from build123d import *

# Parameters (mm, degrees)
F1_DEPTH = 20


with BuildPart() as f1:
    # F0 (on Front) → F1 (new body)
    with BuildSketch(Plane.XZ):
        with BuildLine():
            Line((550, 0), (50, 0))
            ThreePointArc((50, 0), (14.644661, -14.644661), (0, -50))
            Line((0, -50), (0, -650))
            ThreePointArc((0, -650), (14.644661, -685.355339), (50, -700))
            Line((50, -700), (296.851258, -700))
            ThreePointArc((296.851258, -700), (317.85788, -695.37314), (334.976714, -682.348872))
            Line((334.976714, -682.348872), (588.125457, -383.994997))
            ThreePointArc((588.125457, -383.994997), (596.93758, -368.875855), (600, -351.646125))
            Line((600, -351.646125), (600, -50))
            ThreePointArc((600, -50), (585.355339, -14.644661), (550, 0))
        make_face()
    extrude(amount=F1_DEPTH)


solid = f1.part
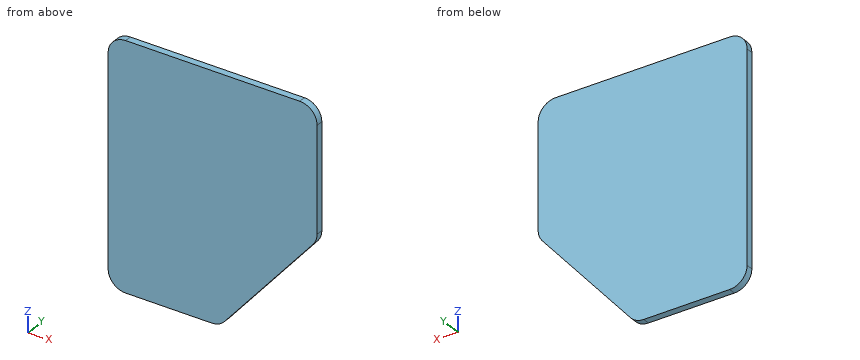
Verification items for the finished model (mm, model axes). Round coordinates to 2 decimals unless told otherwise and drop trailing zeros. Loops run counter-clockwise (first coordinate to the right, second up) from the corner with the lowest first, then second, coordinate; pieces in that order, holes last. Notation, with made-up numbers: (48, 67) - (69, 67) arc R14 cw to (69, 77) - close; hole circle Ø5 at (1.25, 58). An arc over 180 degrees is marked (long way). Answer in a Markdown table with one row per item. Add a question column.
Q1. Section check C-C on z = -565. Enter the section's corners in (x, y).
Q2. Section check A-A on y = -6.75. Enter the section's corners in (x, z) (3 decimals), plus the area to 3 significant figures.
Q3. Material ranges on line 1 (Z direction, x = 298, y = -1); line 2 (X direction, y = -17.5, z = -476); line 3 (Z direction, x = 364.5, y = -9.5), recorded low to high.
Q4. Section check B-B on z = -450. Enter the section's corners in (x, y), plus the area to 3 significant figures.
Found:
| question | item | result |
|---|---|---|
| 1 | outline | (0, -20) - (434.55, -20) - (434.55, 0) - (0, 0) - close |
| 2 | outline | (0, -650) arc R50 ccw to (50, -700) - (296.851, -700) arc R50 ccw to (334.977, -682.349) - (588.125, -383.995) arc R50 ccw to (600, -351.646) - (600, -50) arc R50 ccw to (550, 0) - (50, 0) arc R50 ccw to (0, -50) - close |
| 2 | area | 372,000 mm² |
| 3 | line 1 | z = -699.99 to 0 |
| 3 | line 2 | x = 0 to 510.06 |
| 3 | line 3 | z = -647.55 to 0 |
| 4 | outline | (0, -20) - (532.12, -20) - (532.12, 0) - (0, 0) - close |
| 4 | area | 10,600 mm² |
